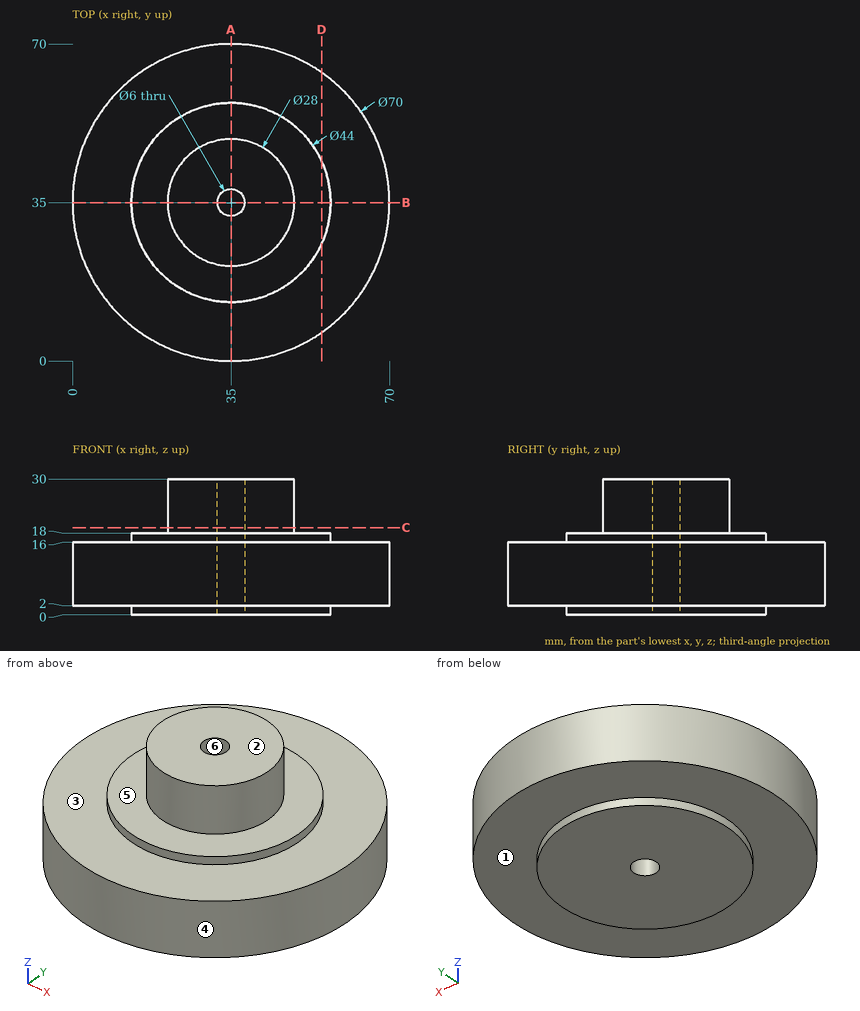
Check sheet for the drawn part. Datum: minimum x, y, z corner. Units: mm. A direction names the side the tool comes from. Coordinates: 2 decimals unless noted, no trailing zeros. Loops run counter-clockwise (first coordinate to the right, second up) from the corner with the lowest first, then second, coordinate; pieces in that order, holes last. Notation, with made-up numbers: M -36.75,12 L -25.75,12 A15 ccw -25.75,21 Z; hole C 7.25,-5.75 d2. An arc over 180 degrees is marked long. Answer as a JSON object with one key per item and string values.
1. Scan lines: L1, parallel to Y at x = 35, z = 13; L2, parallel to Y at x = 35, z = 19.5; L3, parallel to Z at x = 24.5, y = 12.5. Record each from-to range of solid material in increasing order. Write a range as from..to.
Outcome:
{"L1": "0..32, 38..70", "L2": "21..32, 38..49", "L3": "2..16"}
2. Sectioned sample at A-A on x = 35. Record the cut outline in (y, z), and give its area (3 significant figures).
Outcome:
{"outline": "M 0,2 L 13,2 L 13,0 L 32,0 L 32,30 L 21,30 L 21,18 L 13,18 L 13,16 L 0,16 Z; M 38,0 L 57,0 L 57,2 L 70,2 L 70,16 L 57,16 L 57,18 L 49,18 L 49,30 L 38,30 Z", "area": "1,310 mm²"}
3. Release check for a two-part mould opening along X. For the marked faces 4, 5 and 6 record: pulls with the +X half, pulls with the -X half, needs draft (parallel to the pull), parting line crosses it, or undercut.
Outcome:
{"face 4": "parting line crosses it", "face 5": "needs draft", "face 6": "undercut"}
4. Access from +Z, -Z, +X, -X, +Y, -Y to the whole of each face (thin tool, end or side, straight path). Record for the marked faces 1, 2 and 3.
Outcome:
{"face 1": "-Z", "face 2": "+Z, +X, -X, +Y, -Y", "face 3": "+Z"}
5. Depth check by flat-ended pin: P1, Ø12, axis at x = 23, z = 21.5, coming from the -Y side; P2, Ø12, axis at y = 14.5, z = 25, coming from the +X side; P3, Ø5, axis at x = 40.5, z = 13.5, coming from the +Y side; P4, Ø1.5, axis at x = 20.5, y = 9.5, coming from the -Z side. Enter the tip coordinate at first touch or a pass-through.
Outcome:
{"P1": "y = 1.34", "P2": "through", "P3": "y = 69.87", "P4": "z = 2"}
6. Sectioned sample at C-C on z = 19.25. Record the cut outline in (x, y).
Outcome:
{"outline": "C 35,35 d28; hole C 35,35 d6"}
7. Sectioned sample at D-D on x = 55. Record the cut outline in (y, z), and give its area (3 significant figures).
Outcome:
{"outline": "M 6.28,2 L 25.83,2 L 25.83,0 L 44.17,0 L 44.17,2 L 63.72,2 L 63.72,16 L 44.17,16 L 44.17,18 L 25.83,18 L 25.83,16 L 6.28,16 Z", "area": "878 mm²"}
